Design review of the part built by this model. Coordinates are the model's own, in mm. A direction names the side the tool comes from. Coordinates: 2 decimals unless noted, no trailing zeros. Write each loop counter-clockwise with the first axis right and the second up, starting at its lowest first coordinate (ties: lowest second). Pieces come first, ordered by that corner, then holes.
Q1. Add section C-C, the plane y = 23. Give the boundary of the cut face in (x, z), plus the area to 3 significant figures.
Q2. Add section A-A, the plane x = 0. Give the boundary of the cut face in (y, z), plus the area to 3 significant figures.
Q3. Machinability: for faces 5 (the face through (-35, 0, 34)), 6 (the face through (0, -35, 34)), 7 (the face through (-33.4, 0.1, 65)), which of the approach directions +Z, -Z, +X, -X, +Y, -Y give a long, thin tool a straight path to every point of the face, cutting with its end or side? Answer none if there is none.
Q4. Clearance check with flat-ended pins moving along their axes: pin 1 Ø3.5 at (x, y) = (-35, -30) entering from +Z; pin 2 Ø1 at (x, z) = (-28.5, 52.5) entering from -Y; pin 3 Ø1.8 at (x, y) = (35, 30) entering from -Z (3 decimals); pin 4 Ø1.5 at (x, z) = (-20.5, 20.5) entering from -Y. State where each tip first meets the part, or that it passes through.
Q5. To check wall thickness, follow probe 1 along Y at (x, z) = (-35, 1); probe 2 along X at (y, z) = (30, 1); probe 3 along X at (y, z) = (0, 41). State the ranges of each line that lie inside material, in increasing order.
Q6. Add section B-B, the plane z = 32. Give the boundary of the cut face in (x, y).
Q7. Add section D-D, the plane x = -15. Give the boundary of the cut face in (y, z).
Q8. The part is to be moulded in two halves that separate along X. For faces 1 (the face through (0, 35, 34)), 2 (the face through (-1, 40, 1)), 3 (the face through (-34.1, -31.2, 1.5)), 4 (the face through (-45, -1, 1)), say which applies: +X half, -X half, draft (parallel to the pull), parting line (faces both ways), or undercut.
Autodesk Inventor part; units mm, degrees
ref_plane "YZ Plane" through (0, 0, 0) normal (1, 0, 0) x (0, 1, 0)
ref_plane "XZ Plane" through (0, 0, 0) normal (0, 1, 0) x (-1, 0, 0)
ref_plane "XY Plane" through (0, 0, 0) normal (0, 0, 1) x (1, 0, 0)
sketch "スケッチ1" plane through (0, 0, 0) normal (0, 0, 1) x (1, 0, 0)
  circle A0 centre (0, 0) radius 35
  circle A1 centre (0, 0) radius 33
  line L0 (-45, 40) -> (45, 40)
  line L1 (45, 40) -> (45, -40)
  line L2 (45, -40) -> (-45, -40)
  line L3 (-45, -40) -> (-45, 40)
  line L4 (-45, 40) -> (45, -40) construction
  line L5 (45, 40) -> (-45, -40) construction
  dimension "d0" = 70
  dimension "d1" = 66
  dimension "d2" = 90
  dimension "d3" = 80
extrude "押し出し1" add sketch "スケッチ1" along normal blind 3 contours L0 L1 L2 L3
sketch "スケッチ2" plane through (0, 0, 3) normal (0, 0, 1) x (1, 0, 0)
  circle A0 centre (0, 0) radius 35
  circle A1 centre (0, 0) radius 35
  circle A2 centre (0, 0) radius 33
  dimension "d6" = 66
extrude "押し出し2" add sketch "スケッチ2" along normal blind 3 and the other way blind 3
sketch "スケッチ3" plane through (0, 0, 6) normal (0, 0, 1) x (1, 0, 0)
  circle A0 centre (0, 0) radius 33
  circle A1 centre (0, 0) radius 35
extrude "押し出し3" add sketch "スケッチ3" along normal blind 59
sketch "スケッチ4" plane through (0, 0, 65) normal (0, 0, 1) x (1, 0, 0)
  circle A0 centre (0, 0) radius 33
  circle A1 centre (0, 0) radius 35
sketch "スケッチ5" plane through (0, 0, 0) normal (0, 0, -1) x (-1, 0, 0)
  line L0 (-45, 40) -> (-35, 40)
  line L1 (-35, 40) -> (-35, 30)
  line L2 (-35, 30) -> (-45, 30)
  line L3 (-45, 30) -> (-45, 40)
  line L4 (-45, -40) -> (-35, -40)
  line L5 (-35, -40) -> (-35, -30)
  line L6 (-35, -30) -> (-45, -30)
  line L7 (-45, -30) -> (-45, -40)
  line L8 (45, -40) -> (35, -40)
  line L9 (35, -40) -> (35, -30)
  line L10 (35, -30) -> (45, -30)
  line L11 (45, -30) -> (45, -40)
  line L12 (45, 40) -> (35, 40)
  line L13 (35, 40) -> (35, 30)
  line L14 (35, 30) -> (45, 30)
  line L15 (45, 30) -> (45, 40)
  dimension "d13" = 10
  dimension "d14" = 10
  dimension "d15" = 10
  dimension "d16" = 10
  dimension "d17" = 10
  dimension "d18" = 10
  dimension "d19" = 10
hole "穴1" at (35, 30, 0) at (-35, 30, 0) at (-35, -30, 0) at (35, -30, 0) direction (0, 0, 1) diameter 3 depth 8 tip angle 118
sketch "スケッチ6" plane through (0, 0, 65) normal (0, 0, 1) x (1, 0, 0)
  circle A0 centre (0, 0) radius 33
  circle A1 centre (0, 0) radius 35
  line L0 (0, 0) -> (28.6703, -20.0752)
  line L1 (0, 0) -> (35, 0) construction
  line L2 (0, 0) -> (20.0752, -28.6703)
  line L3 (0, 0) -> (35, 0) construction
  line L4 (0, 0) -> (-20.0752, -28.6703)
  line L5 (0, 0) -> (-28.6703, -20.0752)
  line L6 (0, 0) -> (-28.6703, 20.0752)
  line L7 (0, 0) -> (-20.0752, 28.6703)
  line L8 (0, 0) -> (20.0752, 28.6703)
  line L9 (0, 0) -> (28.6703, 20.0752)
  arc A2 (-20.0752, 28.6703) -> (-28.6703, 20.0752) centre (0, 0) ccw
  arc A3 (-18.928, 27.032) -> (-27.032, 18.928) centre (0, 0) ccw
  arc A4 (-27.032, -18.928) -> (-18.928, -27.032) centre (0, 0) ccw
  arc A5 (-28.6703, -20.0752) -> (-20.0752, -28.6703) centre (0, 0) ccw
  arc A6 (18.928, -27.032) -> (27.032, -18.928) centre (0, 0) ccw
  arc A7 (27.032, 18.928) -> (18.928, 27.032) centre (0, 0) ccw
  arc A8 (20.0752, -28.6703) -> (28.6703, -20.0752) centre (0, 0) ccw
  arc A9 (28.6703, 20.0752) -> (20.0752, 28.6703) centre (0, 0) ccw
  dimension "d27" = 35
  dimension "d28" = 55
  dimension "d31" = 360
extrude "押し出し4" cut sketch "スケッチ6" against normal blind 62 contours A0 L8 A1 L9 | L0 A1 L2 A0 | A0 L6 A1 L7 | L4 A1 L5 A0
properties part number "知能ロボコン発射口ver2.1"
Here are the results:
1. outline: (-45, 0) - (-23.66, 0) - (-23.66, 3) - (-45, 3) - close; (23.66, 0) - (45, 0) - (45, 3) - (23.66, 3) - close
1. area: 128 mm2
2. outline: (-40, 0) - (-33, 0) - (-33, 65) - (-35, 65) - (-35, 3) - (-40, 3) - close; (33, 0) - (40, 0) - (40, 3) - (35, 3) - (35, 65) - (33, 65) - close
2. area: 290 mm2
3. face 5: +Z, -X
3. face 6: +Z, -Y
3. face 7: +Z, +X, -X, +Y, -Y
4. pin 1: stops at z = 3
4. pin 2: stops at y = -20.08
4. pin 3: passes through
4. pin 4: stops at y = -28.9
5. probe 1: y = -40 to -31.5, -28.5 to 28.5, 31.5 to 40
5. probe 2: x = -45 to -36.5, -33.5 to -13.75, 13.75 to 33.5, 36.5 to 45
5. probe 3: x = -35 to -33, 33 to 35
6. outline: (-28.67, -20.08) - (-27.03, -18.93) arc R33 cw to (-27.03, 18.93) - (-28.67, 20.08) arc R35 ccw to start; (-20.08, -28.67) arc R35 ccw to (20.08, -28.67) - (18.93, -27.03) arc R33 cw to (-18.93, -27.03) - close; (-20.08, 28.67) - (-18.93, 27.03) arc R33 cw to (18.93, 27.03) - (20.08, 28.67) arc R35 ccw to start; (27.03, -18.93) - (28.67, -20.08) arc R35 ccw to (28.67, 20.08) - (27.03, 18.93) arc R33 cw to start
7. outline: (-40, 0) - (-29.39, 0) - (-29.39, 65) - (-31.62, 65) - (-31.62, 3) - (-40, 3) - close; (29.39, 0) - (40, 0) - (40, 3) - (31.62, 3) - (31.62, 65) - (29.39, 65) - close
8. face 1: parting line
8. face 2: draft
8. face 3: undercut
8. face 4: -X half
